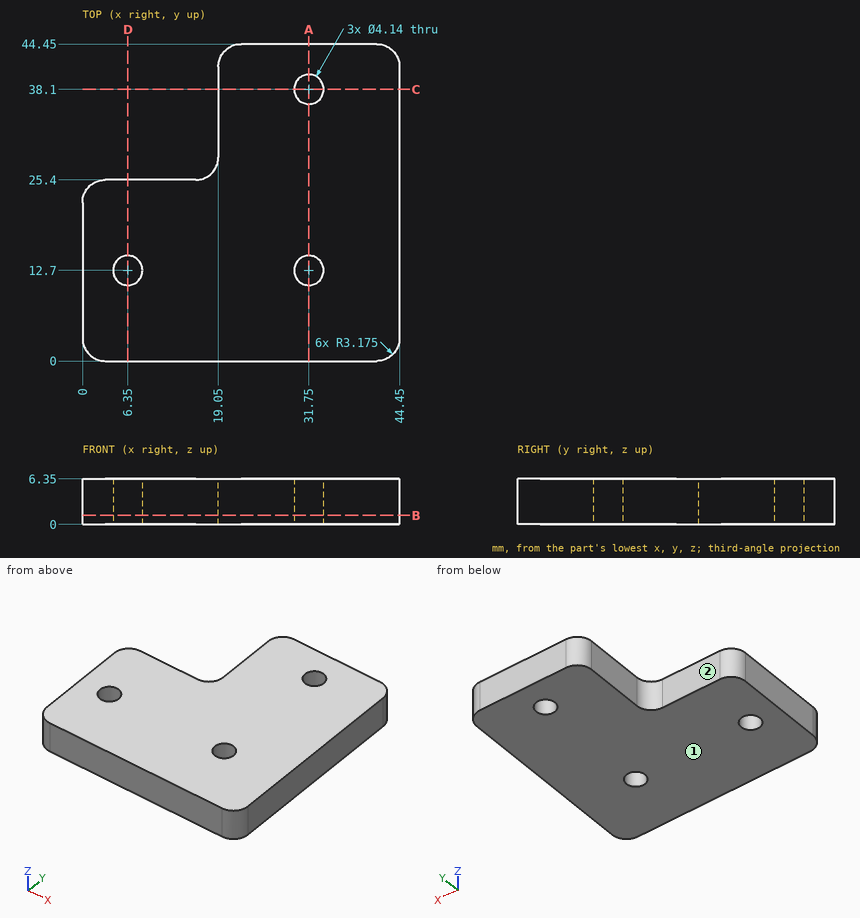
Design review of the part shown in the three views and the two pictorial views. Dimensions are in mm from the part's minimum x, y and z. A direction names the side the tool comes from. Give positions to 0.01 mm unless a question says otherwise; leave off trailing zeros. Write each loop counter-clockwise with the first axis right and the second up, starting at its lowest first coordinate (ties: lowest second). Pieces come first, ordered by that corner, then holes. Notation, with made-up numbers: (72, -9.75) -> (126, -9.75) arc R16 cw to (126, -0.75) -> close; hole circle Ø10 at (-40, 59). An arc over 180 degrees is marked (long way). Answer in a Markdown table with one row per item.
1) Add section C-C on y = 38.1. State the section outline as (x, z) points.
Worked answers:
| item | result |
|---|---|
| outline | (19.05, 0) -> (29.68, 0) -> (29.68, 6.35) -> (19.05, 6.35) -> close; (33.82, 0) -> (44.45, 0) -> (44.45, 6.35) -> (33.82, 6.35) -> close |
2) Clearance check with flat-ended pins moving along their axes: P1, Ø2.5, axis at x = 6.35, y = 12.7, coming from the -Z side; P2, Ø1, axis at x = 9, z = 4, coming from the +Y side. State where each tip first meets the part, or that it passes through.
Worked answers:
| item | result |
|---|---|
| P1 | through |
| P2 | y = 25.4 |
3) Add section A-A on x = 31.75. State the section outline as (y, z) points, plus the area to 3 significant figures.
Worked answers:
| item | result |
|---|---|
| outline | (0, 0) -> (10.63, 0) -> (10.63, 6.35) -> (0, 6.35) -> close; (14.77, 0) -> (36.03, 0) -> (36.03, 6.35) -> (14.77, 6.35) -> close; (40.17, 0) -> (44.45, 0) -> (44.45, 6.35) -> (40.17, 6.35) -> close |
| area | 230 mm² |
4) Add section D-D on x = 6.35. State the section outline as (y, z) points.
Worked answers:
| item | result |
|---|---|
| outline | (0, 0) -> (10.63, 0) -> (10.63, 6.35) -> (0, 6.35) -> close; (14.77, 0) -> (25.4, 0) -> (25.4, 6.35) -> (14.77, 6.35) -> close |
5) For L1, parallel to Y at x = 31.75, z = 4; L2, parallel to Y at x = 6.35, z = 4.75; L3, parallel to Y at x = 16, z = 3.5, list the stretches that pass through material, from the lowest coordinate up. Write a range as [from, to].
Worked answers:
| item | result |
|---|---|
| L1 | [0, 10.63], [14.77, 36.03], [40.17, 44.45] |
| L2 | [0, 10.63], [14.77, 25.4] |
| L3 | [0, 25.4] |
6) Add section B-B on z = 1.25. Count the separate pieces of the cut face and the enclosed holes in it, plus the area to 3 significant figures.
Worked answers:
| item | result |
|---|---|
| separate pieces | 1 |
| enclosed holes | 3 |
| area | 1,560 mm² |
7) Tool access review of the marked faces 1 and 2: name each direction out of +Z, -Z, +X, -X, +Y, -Y from which nothing blocks a thin tool from reaching the whole face with its end or side.
Worked answers:
| item | result |
|---|---|
| face 1 | -Z, +X, -X, +Y, -Y |
| face 2 | +Z, -Z, -X, +Y |
